The listing builds one solid part. Answer for the finished solid, in the listing's coordinates (mm). Face numbers are marked on the shaded views. A direction names the side the tool comes from. Give positions to 0.01 mm unless a question says otherwise; leave off trailing zeros. Loops run counter-clockwise (first coordinate to the right, second up) from the corner with the lowest first, then second, coordinate; pieces in that order, holes last.
Item 1: Section B-B, the plane x = -4.5 is taken. Give the number of separate pieces and of enclosed holes in the cut face, and give its area (3 significant figures).
Item 2: A tool of negligible diameter and unlimited length cuts with its end or side. For the marked faces 4 and 5, from which of +Z, -Z, +X, -X, +Y, -Y can it reach the whole face along a straight path? Write none if from no direction.
Item 3: The mould has two halves that part along X. Classify the marked faces 1, 2 and 3: pulls with the +X half, pulls with the -X half, needs draft (parallel to the pull), parting line crosses it, or undercut.
Item 4: Consider line 1 along Z through (x, y) = (10.5, 31.5) (3 decimals); line 2 along Y through (x, z) = (0, -3.25) (3 decimals). Determine where each line is inside the solid, lowest interval first.
Item 5: Section A-A, the plane z = 4 is taken. Give the vertices of the cut face in (x, y) (3 decimals), and give its area (3 significant figures).
Item 6: Each of these flat-tipped pins is pushed along its axis until it touches: pin 1 Ø1.8 at (x, y) = (15.24, 25.4) entering from +Z; pin 2 Ø3.5 at (x, z) = (1, 5.5) entering from -Y; pin 3 Ø6 at (y, z) = (43.5, 0) entering from +X; pin 4 Ø5 at (y, z) = (18, 0.5) entering from +X. Where does it stop, or does it pass through?
from build123d import *

# Parameters (mm, degrees)
SHELL1_T                    = -6.35
CUT_EXTRUDE1_LETTER_A_DEPTH = 134.19872387
SKETCH4_R                   = 6.35
CUT_EXTRUDE2_AXLE_DEPTH     = 134.19872387
SCALE1_SCALE                = 0.5
SKETCH5_R                   = 0.762
CUT_EXTRUDE1_DEPTH          = 67.599362011


with BuildPart() as part:
    # Sketch2 → Loft1 section 0
    with BuildSketch(Plane(origin=(0, 114.3, 0), x_dir=(1, 0, 0), z_dir=(0, 1, 0))):
        with BuildLine():
            Line((-6.35, -12.7), (6.35, -12.7))
            Line((6.35, -12.7), (6.35, 12.7))
            Line((6.35, 12.7), (-6.35, 12.7))
            Line((-6.35, 12.7), (-6.35, -12.7))
        make_face()
    # Sketch1 → Loft1 section 1
    with BuildSketch(Plane(origin=(0, 0, 0), x_dir=(1, 0, 0), z_dir=(0, 1, 0))):
        with BuildLine():
            Line((-63.5, -12.7), (63.5, -12.7))
            Line((63.5, -12.7), (63.5, 12.7))
            Line((63.5, 12.7), (-63.5, 12.7))
            Line((-63.5, 12.7), (-63.5, -12.7))
        make_face()
    loft()

    # Shell1
    shell1_openings = [part.faces().sort_by_distance(p)[0] for p in [
        (0, 0, 0),
    ]]
    offset(amount=SHELL1_T, openings=shell1_openings, kind=Kind.INTERSECTION)

    # Sketch3 → Cut-Extrude1 Letter A (cut, through all)
    with BuildSketch(Plane.XY.offset(12.7)):
        Polygon((6.35, 91.44), (22.86, 55.88), (-22.86, 55.88), (-6.35, 91.44), align=None)
        Polygon((28.302857143, 45.72), (49.53, 0), (-48.804285714, 0), (-27.577142857, 45.72), align=None)
    extrude(amount=-CUT_EXTRUDE1_LETTER_A_DEPTH, mode=Mode.SUBTRACT)

    # Sketch4 → Cut-Extrude2 Axle (cut, through all)
    with BuildSketch(Plane.XY.offset(12.7)):
        with Locations((0, 101.6)):
            Circle(SKETCH4_R)
    extrude(amount=-CUT_EXTRUDE2_AXLE_DEPTH, mode=Mode.SUBTRACT)


with BuildPart() as part_1:
    # Scale1: scaled about (0, 0, 0)
    add(part.part.scale(SCALE1_SCALE))

    # Sketch5 → Cut-Extrude1 (cut, through all)
    with BuildSketch(Plane.XY.offset(6.35)):
        with Locations((-15.24, 25.4)):
            Circle(SKETCH5_R)
        with Locations(Location((15.24, 25.4, 0), (0, 0, 90))):
            Circle(SKETCH5_R)
    extrude(amount=-CUT_EXTRUDE1_DEPTH, mode=Mode.SUBTRACT)


solid = part_1.part
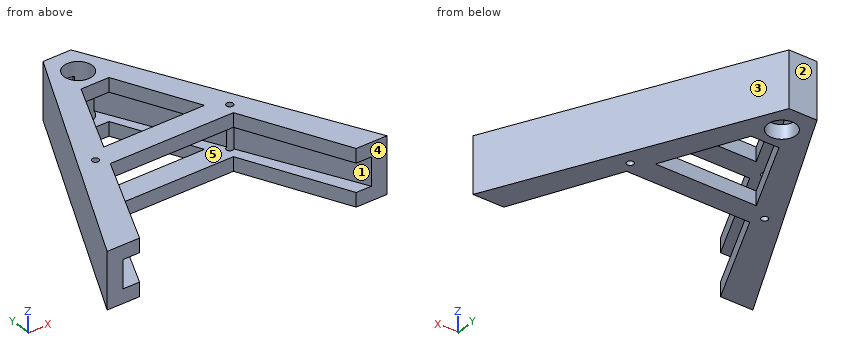
Worked answers:
1. separate pieces: 3
1. enclosed holes: 0
1. area: 151 mm2
2. face 4: +Z, -Z, +X, -X, -Y
2. face 5: -Y
3. face 1: undercut
3. face 2: needs draft
3. face 3: pulls with the +X half
4. line 1: z = -6.35 to -3.175, 3.175 to 6.35
4. line 2: y = 22.86 to 27.94, 45.72 to 47.625, 53.975 to 57.15
5. outline: (-31.75, 0) - (-24.402, 0) - (-13.789, 22.86) - (14.151, 22.86) - (24.765, 0) - (31.75, 0) - (3.175, 57.15) - (-3.175, 57.15) - close; hole circle Ø1.524 at (-15.24, 25.4); hole (-11.43, 27.94) - (11.43, 27.94) - (3.175, 45.72) - (-3.175, 45.72) - close; hole circle Ø6.35 at (0, 50.8); hole circle Ø1.524 at (15.24, 25.4)
5. area: 820 mm2
6. pin 1: stops at z = 6.35
6. pin 2: stops at y = 22.86
6. pin 3: stops at x = 11.5
6. pin 4: stops at x = 24
